```python
from build123d import *

# Parameters (mm, degrees)
SHELL1_T           = 2
SKETCH2_R          = 125.720178412
CUT_EXTRUDE1_DEPTH = 156
SKETCH3_R          = 99
CUT_EXTRUDE2_DEPTH = 4


with BuildPart() as part:
    # Sketch1 → Revolve1 (revolve)
    with BuildSketch(Plane(origin=(0, 0, 0), x_dir=(1, 0, 0), z_dir=(0, 1, 0))):
        with BuildLine():
            Line((0, 100), (0, -100))
            ThreePointArc((0, -100), (100, 0), (0, 100))
        make_face()
    revolve(axis=Axis((0, 0, -100), (0, 0, 1)))

    # Shell1 (no face opened: a closed hollow body)
    add(offset(amount=-SHELL1_T, mode=Mode.PRIVATE), mode=Mode.SUBTRACT)

    # Sketch2 → Cut-Extrude1 (cut)
    with BuildSketch(Plane(origin=(0, 0, 0), x_dir=(1, 0, 0), z_dir=(0, 1, 0))):
        Circle(SKETCH2_R)
    extrude(amount=-CUT_EXTRUDE1_DEPTH, mode=Mode.SUBTRACT)

    # Sketch3 → Cut-Extrude2 (cut)
    with BuildSketch(Plane(origin=(0, 0, 0), x_dir=(-1, 0, 0), z_dir=(0, -1, 0))):
        with Locations(Location((0, 0, 0), (0, 0, 90))):
            Circle(SKETCH3_R)
    extrude(amount=-CUT_EXTRUDE2_DEPTH, mode=Mode.SUBTRACT)


solid = part.part
```
The model under review builds one solid part; all positions refer to its coordinate system, in mm. Round coordinates to 2 decimals unless told otherwise and drop trailing zeros. Order: outer loops, then holes, each group sorted by start corner. A loop starts at its lowest first (then second) coordinate and runs counter-clockwise, first axis right, second up.
(1) Take a section at B-B, the plane z = 0. State the section outline as (x, y) points, plus the area to 3 significant figures.
Working result:
outline: (-100, 0) - (-99, 0) - (-99, 4) - (-97.92, 4) arc R98 cw to (97.92, 4) - (99, 4) - (99, 0) - (100, 0) arc R100 ccw to start
area: 614 mm2
(2) Mouldability with a two-part tool opening along Z and no side actions: class faces 1 (the face through (-97, 0, -23)), 2 (the face through (66.909, 1.972, 72.967)) as released by +Z, released by -Z, zero draft, split by the parting line, or undercut.
Working result:
face 1: zero draft
face 2: undercut
(3) Take a section at C-C, the plane y = 63. State the section outline as (x, z) points.
Working result:
outline: circle Ø155.32 at (0, 0); hole circle Ø150.13 at (0, 0)
(4) Take a section at A-A, the plane x = 0. State the section outline as (y, z) points, plus the area to 3 significant figures.
Working result:
outline: (0, -100) arc R100 ccw to (0, 100) - (0, 99) - (4, 99) - (4, 97.92) arc R98 cw to (4, -97.92) - (4, -99) - (0, -99) - close
area: 614 mm2
(5) For P1, Ø4, axis at x = -60.5, y = 20.5, coming from the +Z side; P2, Ø3, axis at x = 1, y = 74, coming from the +Z side; P3, Ø2, axis at x = 18.5, y = 10.5, coming from the -Z side, all flat-tipped, find the tip position at first contact; note any pin that passes through.
Working result:
P1: stops at z = 78.56
P2: stops at z = 68.87
P3: stops at z = -97.92
(6) Wall thickness on L1, parallel to X at y = 1, z = 0 (3 decimals); L2, parallel to X at y = 19, z = -72.5; L3, parallel to Z at x = -1, y = 64: over which ranges is each line inside the solid? List them lowest first.
Working result:
L1: x = -99.995 to -99, 99 to 99.995
L2: x = -66.2 to -63.14, 63.14 to 66.2
L3: z = -76.83 to -74.21, 74.21 to 76.83
